```python
from build123d import *

# Parameters (mm, degrees)
ESQUISSE1_W             = 45
ESQUISSE1_H             = 45
ESQUISSE1_R             = 1.5
EXTRUSION1_DEPTH        = 5
ESQUISSE2_W             = 45
ESQUISSE2_H             = 5
EXTRUSION2_DEPTH        = 95
EXTRUSION3_DEPTH        = 5
ESQUISSE4_W             = 95
ESQUISSE4_H             = 40
EXTRUSION4_DEPTH        = 5
ESQUISSE5_W             = 100
ESQUISSE5_H             = 5
EXTRUSION5_DEPTH        = 40
ESQUISSE6_W             = 40
ESQUISSE6_H             = 40
EXTRUSION6_DEPTH        = 5
EXTRUSION7_DEPTH        = 5
ENL_V_MAT_EXTRU_1_REACH = 102
ESQUISSE8_R             = 1.5
ENL_V_MAT_EXTRU_2_REACH = 7
ESQUISSE9_R             = 1.5
ESQUISSE10_W            = 88.935907412
ESQUISSE10_H            = 49.014601793
ENL_V_MAT_EXTRU_3_DEPTH = 45
ESQUISSE11_W            = 62.142779394
ESQUISSE11_H            = 38.028527447
ENL_V_MAT_EXTRU_4_DEPTH = 40
ENL_V_MAT_EXTRU_5_REACH = 7
ESQUISSE12_R            = 2


with BuildPart() as part:
    # Esquisse1 → Extrusion1 (new body)
    with BuildSketch(Plane.XY):
        with Locations((22.5, 22.5)):
            Rectangle(ESQUISSE1_W, ESQUISSE1_H)
        with Locations((31.692388155, 31.692388155)):
            Circle(ESQUISSE1_R, mode=Mode.SUBTRACT)
        with Locations((31.692388155, 13.307611845)):
            Circle(ESQUISSE1_R, mode=Mode.SUBTRACT)
        with Locations((13.307611845, 13.307611845)):
            Circle(ESQUISSE1_R, mode=Mode.SUBTRACT)
        with Locations((13.307611845, 31.692388155)):
            Circle(ESQUISSE1_R, mode=Mode.SUBTRACT)
        with BuildLine():
            Line((13.5, 26.858898944), (13.5, 18.141101056))
            ThreePointArc((13.5, 18.141101056), (22.5, 12.5), (31.5, 18.141101056))
            Line((31.5, 18.141101056), (31.5, 26.858898944))
            ThreePointArc((31.5, 26.858898944), (22.5, 32.5), (13.5, 26.858898944))
        make_face(mode=Mode.SUBTRACT)
    extrude(amount=EXTRUSION1_DEPTH)

    # Esquisse2 → Extrusion2 (add)
    with BuildSketch(Plane.XY.offset(5)):
        with Locations((22.5, 2.5)):
            Rectangle(ESQUISSE2_W, ESQUISSE2_H)
    extrude(amount=EXTRUSION2_DEPTH)

    # Esquisse3 → Extrusion3 (add)
    with BuildSketch(Plane(origin=(45, 0, 0), x_dir=(0, 0, -1), z_dir=(1, 0, 0))):
        Polygon((-5, 5), (-5, 45), (-50, 5), align=None)
    extrude(amount=-EXTRUSION3_DEPTH)

    # Esquisse4 → Extrusion4 (add)
    with BuildSketch(Plane.ZY):
        with Locations((52.5, 25)):
            Rectangle(ESQUISSE4_W, ESQUISSE4_H)
    extrude(amount=-EXTRUSION4_DEPTH)

    # Esquisse5 → Extrusion5 (add)
    with BuildSketch(Plane.ZY):
        with Locations((50, 2.5)):
            Rectangle(ESQUISSE5_W, ESQUISSE5_H)
    extrude(amount=EXTRUSION5_DEPTH)

    # Esquisse6 → Extrusion6 (add)
    with BuildSketch(Plane.XY.offset(100)):
        with Locations((-20, 25)):
            Rectangle(ESQUISSE6_W, ESQUISSE6_H)
    extrude(amount=-EXTRUSION6_DEPTH)

    # Esquisse7 → Extrusion7 (add)
    with BuildSketch(Plane.ZY.offset(40)):
        Polygon((95, 5), (95, 45), (50, 5), align=None)
    extrude(amount=-EXTRUSION7_DEPTH)

    # Esquisse8 → Enlèv. mat.-Extru.1 (cut, up to next)
    with BuildSketch(Plane.XY.offset(100), mode=Mode.PRIVATE) as enl_v_mat_extru_1_sk1:
        with Locations((-26.692388155, 31.692388155)):
            Circle(ESQUISSE8_R)
    enl_v_mat_extru_1_tool1 = extrude(enl_v_mat_extru_1_sk1.sketch, amount=-ENL_V_MAT_EXTRU_1_REACH, mode=Mode.PRIVATE) & part.part
    add(enl_v_mat_extru_1_tool1.solids().sort_by_distance((-26.692388, 31.692388, 100))[0], mode=Mode.SUBTRACT)
    # Esquisse8 → Enlèv. mat.-Extru.1 (cut, up to next)
    with BuildSketch(Plane.XY.offset(100), mode=Mode.PRIVATE) as enl_v_mat_extru_1_sk2:
        with Locations((-26.692388155, 13.307611845)):
            Circle(ESQUISSE8_R)
    enl_v_mat_extru_1_tool2 = extrude(enl_v_mat_extru_1_sk2.sketch, amount=-ENL_V_MAT_EXTRU_1_REACH, mode=Mode.PRIVATE) & part.part
    add(enl_v_mat_extru_1_tool2.solids().sort_by_distance((-26.692388, 13.307612, 100))[0], mode=Mode.SUBTRACT)
    # Esquisse8 → Enlèv. mat.-Extru.1 (cut, up to next)
    with BuildSketch(Plane.XY.offset(100), mode=Mode.PRIVATE) as enl_v_mat_extru_1_sk3:
        with Locations((-8.307611845, 13.307611845)):
            Circle(ESQUISSE8_R)
    enl_v_mat_extru_1_tool3 = extrude(enl_v_mat_extru_1_sk3.sketch, amount=-ENL_V_MAT_EXTRU_1_REACH, mode=Mode.PRIVATE) & part.part
    add(enl_v_mat_extru_1_tool3.solids().sort_by_distance((-8.307612, 13.307612, 100))[0], mode=Mode.SUBTRACT)
    # Esquisse8 → Enlèv. mat.-Extru.1 (cut, up to next)
    with BuildSketch(Plane.XY.offset(100), mode=Mode.PRIVATE) as enl_v_mat_extru_1_sk4:
        with Locations((-8.307611845, 31.692388155)):
            Circle(ESQUISSE8_R)
    enl_v_mat_extru_1_tool4 = extrude(enl_v_mat_extru_1_sk4.sketch, amount=-ENL_V_MAT_EXTRU_1_REACH, mode=Mode.PRIVATE) & part.part
    add(enl_v_mat_extru_1_tool4.solids().sort_by_distance((-8.307612, 31.692388, 100))[0], mode=Mode.SUBTRACT)
    # Esquisse8 → Enlèv. mat.-Extru.1 (cut, up to next)
    with BuildSketch(Plane.XY.offset(100), mode=Mode.PRIVATE) as enl_v_mat_extru_1_sk5:
        with BuildLine():
            Line((-26.5, 18.141101056), (-26.5, 26.858898944))
            ThreePointArc((-26.5, 26.858898944), (-17.5, 32.5), (-8.5, 26.858898944))
            Line((-8.5, 26.858898944), (-8.5, 18.141101056))
            ThreePointArc((-8.5, 18.141101056), (-17.5, 12.5), (-26.5, 18.141101056))
        make_face()
    enl_v_mat_extru_1_tool5 = extrude(enl_v_mat_extru_1_sk5.sketch, amount=-ENL_V_MAT_EXTRU_1_REACH, mode=Mode.PRIVATE) & part.part
    add(enl_v_mat_extru_1_tool5.solids().sort_by_distance((-17.5, 22.5, 100))[0], mode=Mode.SUBTRACT)

    # Esquisse9 → Enlèv. mat.-Extru.2 (cut, up to next)
    with BuildSketch(Plane(origin=(0, 5, 0), x_dir=(-1, 0, 0), z_dir=(0, 1, 0)), mode=Mode.PRIVATE) as enl_v_mat_extru_2_sk1:
        with Locations((-40, 95)):
            Circle(ESQUISSE9_R)
    enl_v_mat_extru_2_tool1 = extrude(enl_v_mat_extru_2_sk1.sketch, amount=-ENL_V_MAT_EXTRU_2_REACH, mode=Mode.PRIVATE) & part.part
    add(enl_v_mat_extru_2_tool1.solids().sort_by_distance((40, 5, 95))[0], mode=Mode.SUBTRACT)
    # Esquisse9 → Enlèv. mat.-Extru.2 (cut, up to next)
    with BuildSketch(Plane(origin=(0, 5, 0), x_dir=(-1, 0, 0), z_dir=(0, 1, 0)), mode=Mode.PRIVATE) as enl_v_mat_extru_2_sk2:
        with Locations((-10, 95)):
            Circle(ESQUISSE9_R)
    enl_v_mat_extru_2_tool2 = extrude(enl_v_mat_extru_2_sk2.sketch, amount=-ENL_V_MAT_EXTRU_2_REACH, mode=Mode.PRIVATE) & part.part
    add(enl_v_mat_extru_2_tool2.solids().sort_by_distance((10, 5, 95))[0], mode=Mode.SUBTRACT)
    # Esquisse9 → Enlèv. mat.-Extru.2 (cut, up to next)
    with BuildSketch(Plane(origin=(0, 5, 0), x_dir=(-1, 0, 0), z_dir=(0, 1, 0)), mode=Mode.PRIVATE) as enl_v_mat_extru_2_sk3:
        with Locations((35, 5)):
            Circle(ESQUISSE9_R)
    enl_v_mat_extru_2_tool3 = extrude(enl_v_mat_extru_2_sk3.sketch, amount=-ENL_V_MAT_EXTRU_2_REACH, mode=Mode.PRIVATE) & part.part
    add(enl_v_mat_extru_2_tool3.solids().sort_by_distance((-35, 5, 5))[0], mode=Mode.SUBTRACT)
    # Esquisse9 → Enlèv. mat.-Extru.2 (cut, up to next)
    with BuildSketch(Plane(origin=(0, 5, 0), x_dir=(-1, 0, 0), z_dir=(0, 1, 0)), mode=Mode.PRIVATE) as enl_v_mat_extru_2_sk4:
        with Locations((5, 5)):
            Circle(ESQUISSE9_R)
    enl_v_mat_extru_2_tool4 = extrude(enl_v_mat_extru_2_sk4.sketch, amount=-ENL_V_MAT_EXTRU_2_REACH, mode=Mode.PRIVATE) & part.part
    add(enl_v_mat_extru_2_tool4.solids().sort_by_distance((-5, 5, 5))[0], mode=Mode.SUBTRACT)
    # Esquisse9 → Enlèv. mat.-Extru.2 (cut, up to next)
    with BuildSketch(Plane(origin=(0, 5, 0), x_dir=(-1, 0, 0), z_dir=(0, 1, 0)), mode=Mode.PRIVATE) as enl_v_mat_extru_2_sk5:
        with Locations((-40, 55)):
            Circle(ESQUISSE9_R)
    enl_v_mat_extru_2_tool5 = extrude(enl_v_mat_extru_2_sk5.sketch, amount=-ENL_V_MAT_EXTRU_2_REACH, mode=Mode.PRIVATE) & part.part
    add(enl_v_mat_extru_2_tool5.solids().sort_by_distance((40, 5, 55))[0], mode=Mode.SUBTRACT)
    # Esquisse9 → Enlèv. mat.-Extru.2 (cut, up to next)
    with BuildSketch(Plane(origin=(0, 5, 0), x_dir=(-1, 0, 0), z_dir=(0, 1, 0)), mode=Mode.PRIVATE) as enl_v_mat_extru_2_sk6:
        with Locations((35, 45)):
            Circle(ESQUISSE9_R)
    enl_v_mat_extru_2_tool6 = extrude(enl_v_mat_extru_2_sk6.sketch, amount=-ENL_V_MAT_EXTRU_2_REACH, mode=Mode.PRIVATE) & part.part
    add(enl_v_mat_extru_2_tool6.solids().sort_by_distance((-35, 5, 45))[0], mode=Mode.SUBTRACT)

    # Esquisse10 → Enlèv. mat.-Extru.3 (cut)
    with BuildSketch(Plane(origin=(0, 0, 0), x_dir=(-1, 0, 0), z_dir=(0, 0, -1))):
        with Locations((-0.532046294, 24.507300897)):
            Rectangle(ESQUISSE10_W, ESQUISSE10_H)
    extrude(amount=-ENL_V_MAT_EXTRU_3_DEPTH, mode=Mode.SUBTRACT)

    # Esquisse11 → Enlèv. mat.-Extru.4 (cut)
    with BuildSketch(Plane(origin=(45, 0, 0), x_dir=(0, 0, -1), z_dir=(1, 0, 0))):
        with Locations((-68.928610303, 19.014263724)):
            Rectangle(ESQUISSE11_W, ESQUISSE11_H)
    extrude(amount=-ENL_V_MAT_EXTRU_4_DEPTH, mode=Mode.SUBTRACT)

    # Esquisse12 → Enlèv. mat.-Extru.5 (cut, up to next)
    with BuildSketch(Plane(origin=(0, 5, 0), x_dir=(-1, 0, 0), z_dir=(0, 1, 0)), mode=Mode.PRIVATE) as enl_v_mat_extru_5_sk1:
        with Locations((19.890130801, 72.49689605)):
            Circle(ESQUISSE12_R)
    enl_v_mat_extru_5_tool1 = extrude(enl_v_mat_extru_5_sk1.sketch, amount=-ENL_V_MAT_EXTRU_5_REACH, mode=Mode.PRIVATE) & part.part
    add(enl_v_mat_extru_5_tool1.solids().sort_by_distance((-19.890131, 5, 72.496896))[0], mode=Mode.SUBTRACT)


solid = part.part
```
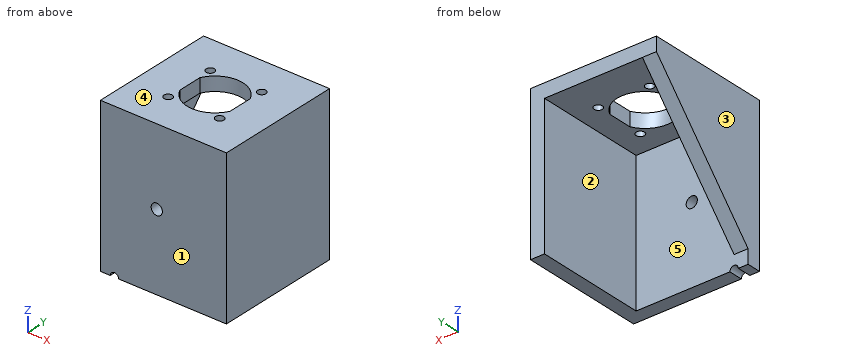
Verification items for the finished model (mm, model axes). Face numbers are marked on the shaded views. A direction names the side the tool comes from. Round coordinates to 2 decimals unless told otherwise and drop trailing zeros. Order: outer loops, then holes, each group sorted by start corner. A loop starts at its lowest first (then second) coordinate and runs counter-clockwise, first axis right, second up. Notation, with made-up numbers: (84.25, 22.5) -> (114.25, 22.5) arc R20 cw to (114.25, 38.5) -> close; hole circle Ø2 at (-31, 28.5). An arc over 180 degrees is marked (long way). Put each result on its own line as item: value. Start each with the question number.
(1) Tool access check on the marked faces 4 and 5. Record the directions out of +Z, -Z, +X, -X, +Y, -Y that give a thin tool (end or side, any length) a straight path to the whole face; none if there is none.
(2) Section check B-B (z = 65.5). Enter the section's corners in (x, y), then the cut area to 3 significant figures.
(3) Section check C-C (y = 39.5). Enter the section's corners in (x, z).
(4) Depth check by flat-ended pin: pin 1 Ø5 at (x, z) = (-19.89, 72.5) entering from +Y; pin 2 Ø2 at (x, y) = (-23.5, 31.5) entering from -Z. Enter the tip coordinate at first touch or a pass-through.
(5) Material ranges on line 1 along X through (y, z) = (22, 74); line 2 along Y through (x, z) = (-17.5, 89.5); line 3 along Z through (x, y) = (-8, 7.5), recorded low to high.
(6) Draft check along X on the marked faces 1, 2 and 3. Enter one of: +X half, -X half, draft (parallel to the pull), parting line (faces both ways), or undercut.
(7) Section check A-A (y = 25). Enter the section's corners in (x, z).
Completed:
1. face 4: +Z, +X, -X, +Y, -Y
1. face 5: -Z, +Y
2. outline: (-40, 0) -> (5, 0) -> (5, 45) -> (0, 45) -> (0, 5) -> (-35, 5) -> (-35, 18.78) -> (-40, 18.78) -> close
2. area: 494 mm2
3. outline: (-40, 88.81) -> (-35, 88.81) -> (-35, 95) -> (0, 95) -> (0, 45) -> (5, 45) -> (5, 100) -> (-40, 100) -> close
4. pin 1: stops at y = 5
4. pin 2: stops at z = 95
5. line 1: x = -40 to -35, 0 to 5
5. line 2: y = 0 to 5
5. line 3: z = 95 to 100
6. face 1: draft
6. face 2: undercut
6. face 3: -X half
7. outline: (-40, 72.5) -> (-35, 72.5) -> (-35, 95) -> (-26.5, 95) -> (-26.5, 100) -> (-40, 100) -> close; (-8.5, 95) -> (0, 95) -> (0, 45) -> (5, 45) -> (5, 100) -> (-8.5, 100) -> close
